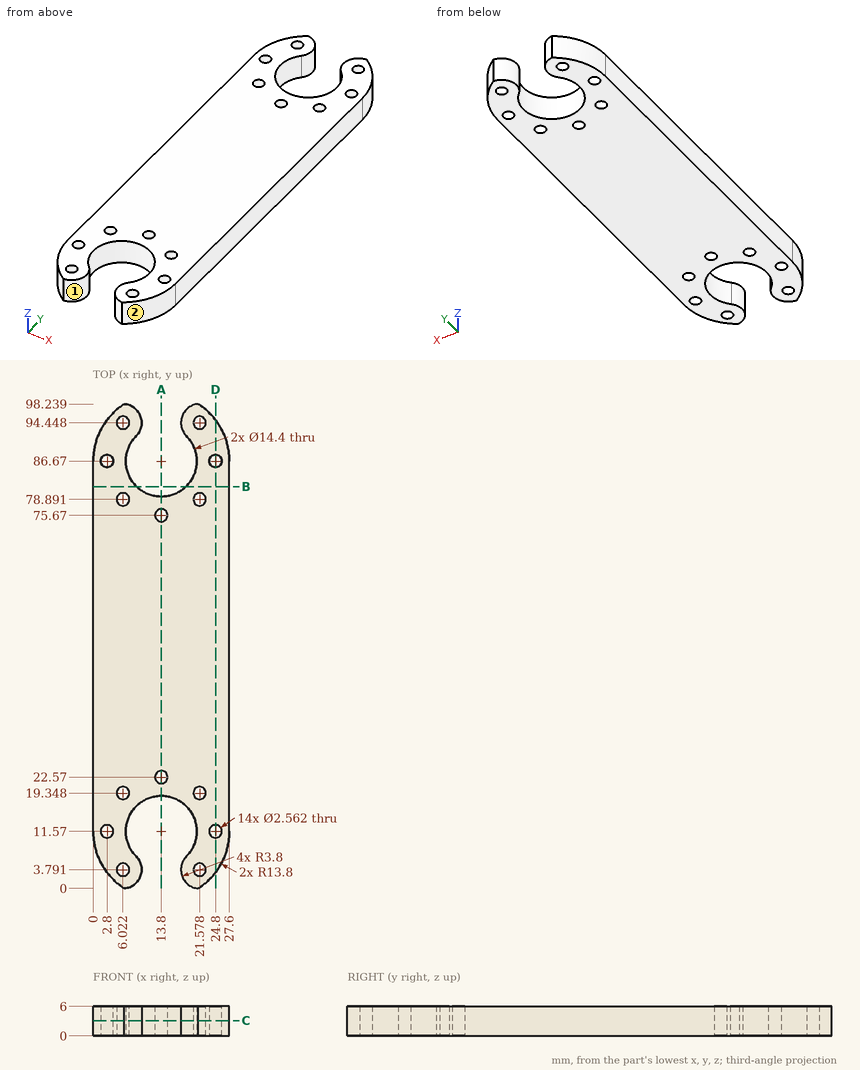
Could you check a few things on this drawing? It's one solid part, dimensions in mm from its lowest x, y, z. A direction names the side the tool comes from. Give positions to 0.01 mm unless a question says otherwise; leave off trailing zeros. Order: outer loops, then holes, each group sorted by start corner. A loop starts at its lowest first (then second) coordinate and runs counter-clockwise, first axis right, second up. Notation, with made-up numbers: M 34.5,-3 L 62.5,-3 A17 ccw 62.5,19 Z; hole C -22,26.25 d9. An arc over 180 degrees is marked long. Use one line per item in the form item = value. Start each with the question number.
Item 1: If we section it at C-C (z = 3.1): State how many separate pieces and enclosed holes the cut face has, then the cut area to 3 significant figures.
Item 2: If I drill on line 1 along Y through (x, z) = (13.8, 1.5); line 2 along Y through (x, z) = (3.25, 1.3) (1 decimal); line 3 along X through (y, z) = (86, 5.6), over which ranges is the centre line in solid material (lowest first)?
Item 3: If we section it at A-A (x = 13.8): Write out the boundary of the cut face in (y, z).
Item 4: If we section it at B-B (y = 81.5): Write out the boundary of the cut face in (x, z).
Item 5: If we section it at D-D (x = 24.8): Write out the boundary of the cut face in (y, z), then the cut area to 3 significant figures.
Item 6: For the marked faces 1 and 2, which set-ups out of +Z, -Z, +X, -X, +Y, -Y let a thin tool reach every point of the face, with its end or its side?
Outcome:
q1.separate_pieces = 1
q1.enclosed_holes = 14
q1.area = 2,140 mm2
q2.line_1 = 18.77 to 21.29, 23.85 to 74.39, 76.95 to 79.47
q2.line_2 = 2.7 to 10.4, 12.8 to 85.5, 87.9 to 95.6
q2.line_3 = 0 to 1.71, 3.89 to 6.63, 20.97 to 23.71, 25.89 to 27.6
q3.outline = M 18.77,0 L 21.29,0 L 21.29,6 L 18.77,6 Z; M 23.85,0 L 74.39,0 L 74.39,6 L 23.85,6 Z; M 76.95,0 L 79.47,0 L 79.47,6 L 76.95,6 Z
q4.outline = M 0,0 L 8.79,0 L 8.79,6 L 0,6 Z; M 18.81,0 L 27.6,0 L 27.6,6 L 18.81,6 Z
q5.outline = M 3.24,0 L 10.29,0 L 10.29,6 L 3.24,6 Z; M 12.85,0 L 85.39,0 L 85.39,6 L 12.85,6 Z; M 87.95,0 L 95,0 L 95,6 L 87.95,6 Z
q5.area = 520 mm2
q6.face_1 = +Z, -Z
q6.face_2 = +Z, -Z, +X, -Y
